Read the model definition and answer for the solid it produces. Units are mm, in the model's axes. A direction names the side the tool comes from. Coordinates: 2 decimals unless noted, no trailing zeros. Write each loop counter-clockwise with the first axis right and the second up, starting at its lowest first coordinate (ties: lowest second). Pieces come first, ordered by that corner, then holes.
Item 1: Section D-D (x = -9) is taken. Give the vertices of the cut face in (y, z).
Item 2: Each of these flat-tipped pins is pushed along its axis until it touches: P1, Ø11.5, axis at x = 1.5, z = 42, coming from the -Y side; P2, Ø4.5, axis at x = -2.5, y = 35.5, coming from the +Z side; P3, Ø13.5, axis at x = 0, z = 35, coming from the -Y side; P4, Ø12, axis at x = 20.5, z = 27, coming from the -Y side. Where does it stop, or does it pass through?
Item 3: Section A-A (x = 0) is taken. Give the vertices of the cut face in (y, z).
Item 4: A tool of negligible diameter and unlimited length cuts with its end or side. For faces 1 (the face through (0, 40, 5)), 2 (the face through (0, 15, 27)), 3 (the face through (0, 1, 0)), 4 (the face through (6, 25, 29)), 5 (the face through (0, -15, 10)), from which of +Z, -Z, +X, -X, +Y, -Y can it reach the whole face along a straight path? Write none if from no direction.
Item 5: Straight lines are drawn through the part: probe 1 along Z at (x, y) = (0, 22); probe 2 along Z at (x, y) = (0, 11); probe 3 along Z at (x, y) = (21.5, -1). For each, find the intervals that lie inside material, in ascending order.
Item 6: Determine the mould class of faces 6 (the face through (-4.119, 12.465, 16.452)), 7 (the face through (-21, 10, 35)), 8 (the face through (-31, 12, 17)) for opening direction X: released by +X, released by -X, zero draft, split by the parting line, or undercut.
Item 7: Section B-B (z = 35) is taken. Give the vertices of the cut face in (x, y), then the cut area to 3 significant figures.
Item 8: Section C-C (y = 20.5) is taken. Give the vertices of the cut face in (x, z).
from build123d import *

# Parameters (mm, degrees)
F0_W     = 62
F0_H     = 15
F1_DEPTH = 60
F0_H_2   = 50
F2_DEPTH = 10
F3_R     = 19
F4_DEPTH = 5
F5_R     = 7.5
F6_DEPTH = 25.001


with BuildPart() as f1:
    # F0 (on Top) → F1 (new body)
    with BuildSketch(Plane.XY):
        with Locations((0, 17.5)):
            Rectangle(F0_W, F0_H)
    extrude(amount=F1_DEPTH)

    # F0 (on Top) → F2 (join)
    with BuildSketch(Plane.XY):
        with Locations((0, 32.5)):
            Rectangle(F0_W, F0_H)
        with Locations((0, -15)):
            Rectangle(F0_W, F0_H_2)
    extrude(amount=F2_DEPTH)

    # F3 (on face) → F4 (cut)
    with BuildSketch(Plane.XZ.offset(-10)):
        with Locations((0, 35)):
            Circle(F3_R)
    extrude(amount=-F4_DEPTH, mode=Mode.SUBTRACT)

    # F5 (on face) → F6 (cut, through all)
    with BuildSketch(Plane.XZ.offset(-15)):
        with Locations((0, 35)):
            Circle(F5_R)
    extrude(amount=-F6_DEPTH, mode=Mode.SUBTRACT)


solid = f1.part
Established:
1. outline: (-40, 0) - (40, 0) - (40, 10) - (25, 10) - (25, 60) - (10, 60) - (10, 51.73) - (15, 51.73) - (15, 18.27) - (10, 18.27) - (10, 10) - (-40, 10) - close
2. P1: stops at y = 15
2. P2: stops at z = 10
2. P3: passes through
2. P4: stops at y = 10
3. outline: (-40, 0) - (40, 0) - (40, 10) - (25, 10) - (25, 27.5) - (15, 27.5) - (15, 16) - (10, 16) - (10, 10) - (-40, 10) - close; (10, 54) - (15, 54) - (15, 42.5) - (25, 42.5) - (25, 60) - (10, 60) - close
4. face 1: +Z, -Z, +X, -X, +Y
4. face 2: -Y
4. face 3: -Z, +X, -X, +Y, -Y
4. face 4: +Z, +X, -X, +Y
4. face 5: +Z, +X, -X, -Y
5. probe 1: z = 0 to 27.5, 42.5 to 60
5. probe 2: z = 0 to 16, 54 to 60
5. probe 3: z = 0 to 10
6. face 6: undercut
6. face 7: zero draft
6. face 8: released by -X
7. outline: (-31, 10) - (-19, 10) - (-19, 15) - (-7.5, 15) - (-7.5, 25) - (-31, 25) - close; (7.5, 15) - (19, 15) - (19, 10) - (31, 10) - (31, 25) - (7.5, 25) - close
7. area: 590 mm2
8. outline: (-31, 0) - (31, 0) - (31, 60) - (-31, 60) - close; hole circle Ø15 at (0, 35)
